The model under review builds one solid part; all positions refer to its coordinate system, in mm. Face numbers are marked on the shaded views. A direction names the side the tool comes from. Round coordinates to 2 decimals unless told otherwise and drop trailing zeros. Loops run counter-clockwise (first coordinate to the right, second up) from the corner with the lowest first, then second, coordinate; pieces in that order, holes last. Notation, with made-up numbers: M -32.5,88 L -22.5,88 A17 ccw -22.5,118 Z; hole C 48,-30 d1. An arc over 180 degrees is marked long. Return JSON: item names as keys, results as strings. Group by question number.
Q1. Draft analysis for pull direction Y (two halves, no side actions). For the marked faces 1, 2 and 3, state which applies: pulls with the +Y half, pulls with the -Y half, needs draft (parallel to the pull), parting line crosses it, or undercut.
Q2. For the marked faces 4 and 5, list the 3-axis set-ups (+Z, -Z, +X, -X, +Y, -Y) from which the entire face can be reached by the end or side of a thin tool; tool diameter is ignored.
Q3. Clearance check with flat-ended pins moving along their axes: pin 1 Ø6 at (x, y) = (-54.5, 12) entering from +Z; pin 2 Ø2 at (y, z) = (20, 17.5) entering from -X; pin 3 Ø2 at (y, z) = (15, 29) entering from +X. State where each tip first meets the part, or that it passes through.
Q4. Consider section B-B (x = -76.5). State the section outline as (y, z) points.
Q5. Consider section D-D (x = -29.5). State the section outline as (y, z) points.
Q6. To check wall thickness, follow line 1 along X through (y, z) = (33, 48); line 2 along X through (y, z) = (14.5, 14); line 3 along Z through (x, y) = (-92, 45.5). State the ranges of each line that lie inside material, in increasing order.
Q7. Consider section C-C (y = 32). State the section outline as (x, z) points, and give its area (3 significant figures).
Q8. Consider section A-A (z = 16). State the section outline as (x, y) points.
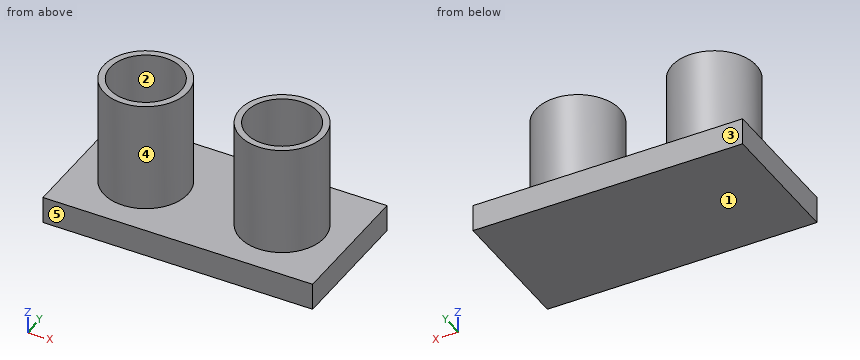
from build123d import *

# Parameters (mm, degrees)
SKETCH1_W           = 100
SKETCH1_H           = 50
BOSS_EXTRUDE1_DEPTH = 10
SKETCH2_R           = 15.587917706
SKETCH2_R_2         = 13.17523912
BOSS_EXTRUDE2_DEPTH = 50.8


with BuildPart() as part:
    # Sketch1 → Boss-Extrude1 (new body)
    with BuildSketch(Plane.XY):
        with Locations((-50, 25)):
            Rectangle(SKETCH1_W, SKETCH1_H)
    extrude(amount=BOSS_EXTRUDE1_DEPTH)

    # Sketch2 → Boss-Extrude2 (add)
    # profile 1 of 2: a face of its own
    with BuildSketch(Plane.XY):
        with Locations((-75.275238724, 24.288037008)):
            Circle(SKETCH2_R)
        with Locations((-75.275238724, 24.288037008)):
            Circle(SKETCH2_R_2, mode=Mode.SUBTRACT)
    # profile 2 of 2: a face of its own
    with BuildSketch(Plane.XY):
        with Locations(Location((-24.724761276, 24.288037008, 0), (0, 0, 180))):
            Circle(SKETCH2_R)
        with Locations(Location((-24.724761276, 24.288037008, 0), (0, 0, 180))):
            Circle(SKETCH2_R_2, mode=Mode.SUBTRACT)
    extrude(amount=BOSS_EXTRUDE2_DEPTH)


solid = part.part
Values:
{
 "1": {"face 1": "needs draft", "face 2": "undercut", "face 3": "pulls with the +Y half"},
 "2": {"face 4": "+Z", "face 5": "+Z, -Z, +X, -X, -Y"},
 "3": {"pin 1": "stops at z = 10", "pin 2": "stops at x = -90.51", "pin 3": "stops at x = -11.52"},
 "4": {"outline": "M 0,0 L 50,0 L 50,10 L 39.83,10 L 39.83,50.8 L 37.41,50.8 L 37.41,10 L 11.17,10 L 11.17,50.8 L 8.75,50.8 L 8.75,10 L 0,10 Z"},
 "5": {"outline": "M 0,0 L 50,0 L 50,10 L 39.13,10 L 39.13,50.8 L 36.57,50.8 L 36.57,10 L 12.01,10 L 12.01,50.8 L 9.45,50.8 L 9.45,10 L 0,10 Z"},
 "6": {"line 1": "x = -88.2 to -85.16, -65.39 to -62.35, -37.65 to -34.61, -14.84 to -11.8", "line 2": "x = -87.41 to -84.09, -66.46 to -63.14, -36.86 to -33.54, -15.91 to -12.59", "line 3": "z = 0 to 10"},
 "7": {"outline": "M -100,0 L 0,0 L 0,10 L -11.18,10 L -11.18,50.8 L -14.04,50.8 L -14.04,10 L -35.41,10 L -35.41,50.8 L -38.27,50.8 L -38.27,10 L -61.73,10 L -61.73,50.8 L -64.59,50.8 L -64.59,10 L -85.96,10 L -85.96,50.8 L -88.82,50.8 L -88.82,10 L -100,10 Z", "area": "1,470 mm2"},
 "8": {"outline": "C -75.28,24.29 d31.18; C -24.72,24.29 d31.18; hole C -75.28,24.29 d26.35; hole C -24.72,24.29 d26.35"}
}
